Work out the finished part from the listing and answer in its coordinate system (mm). A direction names the side the tool comes from. Round coordinates to 2 decimals unless told otherwise and drop trailing zeros. Loops run counter-clockwise (first coordinate to the right, second up) from the corner with the lowest first, then second, coordinate; pieces in that order, holes last.
```python
from build123d import *

# Parameters (mm, degrees)
SKETCH_1_R          = 3.45
EXTRUDE_1_DEPTH     = 23
CUT_EXTRUDE_1_DEPTH = 5.5
SKETCH_3_R          = 4
EXTRUDE_2_DEPTH     = 2
SKETCH_4_R          = 17.5
EXTRUDE_3_DEPTH     = 4
CUT_EXTRUDE_2_DEPTH = 3
SKETCH_6_R          = 1.75
CUT_EXTRUDE_3_DEPTH = 2
FILLET_1_R          = 0.5
FILLET_2_R          = 1


with BuildPart() as part:
    # Эскиз1 → Бобышка-Вытянуть1 (new body)
    with BuildSketch(Plane(origin=(0, 0, 0), x_dir=(1, 0, 0), z_dir=(0, 1, 0))):
        Circle(SKETCH_1_R)
    extrude(amount=EXTRUDE_1_DEPTH)

    # Эскиз2 → Вырез-Вытянуть1 (cut)
    with BuildSketch(Plane.XZ):
        with BuildLine():
            Line((-1.55, 2.391652149), (-1.55, -2.391652149))
            ThreePointArc((-1.55, -2.391652149), (0, -2.85), (1.55, -2.391652149))
            Line((1.55, -2.391652149), (1.55, 2.391652149))
            ThreePointArc((1.55, 2.391652149), (0, 2.85), (-1.55, 2.391652149))
        make_face()
    extrude(amount=-CUT_EXTRUDE_1_DEPTH, mode=Mode.SUBTRACT)

    # Эскиз3 → Бобышка-Вытянуть2 (add)
    with BuildSketch(Plane(origin=(0, 23, 0), x_dir=(1, 0, 0), z_dir=(0, 1, 0))):
        Circle(SKETCH_3_R)
    extrude(amount=EXTRUDE_2_DEPTH)

    # Эскиз4 → Бобышка-Вытянуть3 (add)
    with BuildSketch(Plane(origin=(0, 25, 0), x_dir=(1, 0, 0), z_dir=(0, 1, 0))):
        Circle(SKETCH_4_R)
    extrude(amount=EXTRUDE_3_DEPTH)

    # Эскиз5 → Вырез-Вытянуть2 (cut)
    with BuildSketch(Plane.XZ.offset(-25)):
        Polygon((13, -3.279349529), (15.84, -1.639674764), (15.84, 1.639674764), (13, 3.279349529), (10.16, 1.639674764), (10.16, -1.639674764), align=None)
        Polygon((3.279349529, 13), (1.639674764, 15.84), (-1.639674764, 15.84), (-3.279349529, 13), (-1.639674764, 10.16), (1.639674764, 10.16), align=None)
        Polygon((-3.279349529, -13), (-1.639674764, -15.84), (1.639674764, -15.84), (3.279349529, -13), (1.639674764, -10.16), (-1.639674764, -10.16), align=None)
        Polygon((-13, 3.279349529), (-15.84, 1.639674764), (-15.84, -1.639674764), (-13, -3.279349529), (-10.16, -1.639674764), (-10.16, 1.639674764), align=None)
    extrude(amount=-CUT_EXTRUDE_2_DEPTH, mode=Mode.SUBTRACT)

    # Эскиз6 → Вырез-Вытянуть3 (cut, through all)
    with BuildSketch(Plane.XZ.offset(-28)):
        with Locations((0, 13)):
            Circle(SKETCH_6_R)
        with Locations((13, 0)):
            Circle(SKETCH_6_R)
        with Locations((0, -13)):
            Circle(SKETCH_6_R)
        with Locations((-13, 0)):
            Circle(SKETCH_6_R)
    extrude(amount=-CUT_EXTRUDE_3_DEPTH, mode=Mode.SUBTRACT)

    # Скругление1
    fillet_1_edges = [part.edges().sort_by_distance(p)[0] for p in [
        (-17.5, 25, 0),
    ]]
    fillet(fillet_1_edges, radius=FILLET_1_R)

    # Скругление2
    fillet_2_edges = [part.edges().sort_by_distance(p)[0] for p in [
        (-4, 25, 0),
    ]]
    fillet(fillet_2_edges, radius=FILLET_2_R)


solid = part.part
```
1. Find section A-A (y = 26.5). Write down the section's boundary in (x, z), then the cut area to 3 significant figures.
Answer key:
outline: circle Ø35 at (0, 0); hole (-15.84, -1.64) - (-13, -3.28) - (-10.16, -1.64) - (-10.16, 1.64) - (-13, 3.28) - (-15.84, 1.64) - close; hole (-3.28, -13) - (-1.64, -15.84) - (1.64, -15.84) - (3.28, -13) - (1.64, -10.16) - (-1.64, -10.16) - close; hole (-3.28, 13) - (-1.64, 10.16) - (1.64, 10.16) - (3.28, 13) - (1.64, 15.84) - (-1.64, 15.84) - close; hole (10.16, -1.64) - (13, -3.28) - (15.84, -1.64) - (15.84, 1.64) - (13, 3.28) - (10.16, 1.64) - close
area: 850 mm2
2. Consider probe 1 along Z at (x, y) = (0, 28.35); probe 2 along Y at (x, z) = (-9.5, 12); probe 3 along Z at (x, y) = (-13, 28.2). Determine where each line is inside the solid, lowest interval first.
Answer key:
probe 1: z = -17.5 to -14.75, -11.25 to 11.25, 14.75 to 17.5
probe 2: y = 25 to 29
probe 3: z = -11.72 to -1.75, 1.75 to 11.72
3. Find section D-D (y = 22). Write down the section's boundary in (x, z), then the cut area to 3 significant figures.
Answer key:
outline: circle Ø6.9 at (0, 0)
area: 37.4 mm2
4. Which of the six approach directions +Z, -Z, +X, -X, +Y, -Y give full straight-line access (tool end or side, diameter ignored) to faces 1 (the face through (2.45, 26.48, 11.56)), 2 (the face through (14.669, 28.493, 0.526))?
Answer key:
face 1: -Y
face 2: +Y, -Y
5. Find section B-B (z = 0). Give the number of separate pieces and of enclosed holes in the cut face, then the cut area to 3 significant figures.
Answer key:
separate pieces: 3
enclosed holes: 0
area: 257 mm2
6. Given pin 1 (2.5 mm diameter, centred on y = 27, z = 0.5, fed in from -X); pin 2 (10 mm diameter, centred on y = 16, z = -12, fed in from -X); pin 3 (2.5 mm diameter, centred on y = 2, z = 0.5, fed in from -X); pin 4 (3 mm diameter, centred on x = -1.5, z = 13, fed in from -Y), each flat-ended and moving along its own axis, determine where each tip first touches the part or whether it passes through.
Answer key:
pin 1: stops at x = -17.5
pin 2: passes through
pin 3: stops at x = -3.45
pin 4: stops at y = 28
7. Determine the mould class of faces 3 (the face through (-13.887, 27.226, 10.648)), 4 (the face through (-0.228, 28.493, -11.265)), 5 (the face through (-3, 23, 2)) for opening direction X: +X half, -X half, draft (parallel to the pull), parting line (faces both ways), or undercut.
Answer key:
face 3: parting line
face 4: undercut
face 5: draft
